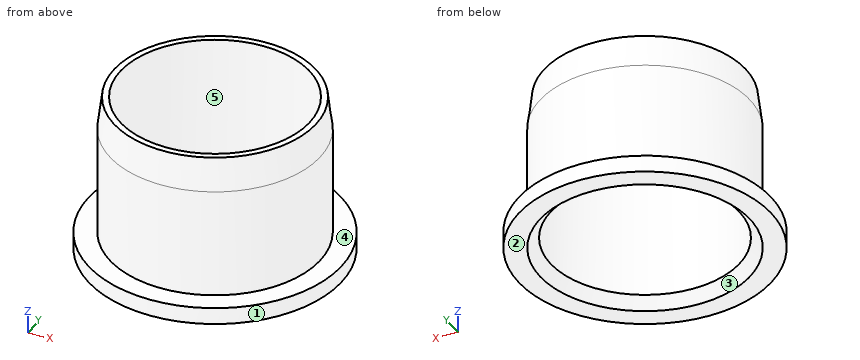
from build123d import *

# Parameters (mm, degrees)
F1_R     = 15.04
F1_R_2   = 12.5
F1_R_3   = 11.25
F2_DEPTH = 2
F3_DEPTH = 17.018
F4_SIZE2 = 4
F4_SIZE  = 0.5
F5_SIZE  = 1.25


with BuildPart() as f2:
    # F1 (on Top) → F2 (new body)
    with BuildSketch(Plane.XY):
        Circle(F1_R)
        Circle(F1_R_2, mode=Mode.SUBTRACT)
        Circle(F1_R_2)
        Circle(F1_R_3, mode=Mode.SUBTRACT)
    extrude(amount=-F2_DEPTH)

    # F1 (on Top) → F3 (join)
    with BuildSketch(Plane.XY):
        Circle(F1_R_2)
        Circle(F1_R_3, mode=Mode.SUBTRACT)
    extrude(amount=F3_DEPTH)

    # F4
    f4_edges = [f2.edges().sort_by_distance(p)[0] for p in [
        (-12.5, 0, 17.018),
    ]]
    f4_side = f2.faces().sort_by_distance((-12.146447, 0, 17.018))[0]
    chamfer(f4_edges, length=F4_SIZE, length2=F4_SIZE2, reference=f4_side)

    # F5
    f5_edges = [f2.edges().sort_by_distance(p)[0] for p in [
        (-11.25, 0, -2),
    ]]
    chamfer(f5_edges, length=F5_SIZE)


solid = f2.part
Work out the finished part from the listing and answer in its coordinate system (mm). Face numbers are marked on the shaded views. A direction names the side the tool comes from. Coordinates: 2 decimals unless noted, no trailing zeros. Write each loop counter-clockwise with the first axis right and the second up, starting at its lowest first coordinate (ties: lowest second). Pieces come first, ordered by that corner, then holes. Notation, with made-up numbers: M 57.25,36.25 L 76.25,36.25 A20 ccw 76.25,44.25 Z; hole C -7,44.5 d6. An arc over 180 degrees is marked long. Write item = value, one per line.
1. Determine the mould class of the marked faces 1, 2 and 3 for opening direction X: released by +X, released by -X, zero draft, split by the parting line, or undercut.
Solution:
face_1 = split by the parting line
face_2 = zero draft
face_3 = undercut
2. Straight lines are drawn through the part: line 1 (Y direction, x = 0, z = 6); line 2 (Y direction, x = 9, z = 1); line 3 (X direction, y = -8, z = 8). For each, find the intervals that lie inside material, in ascending order. Write a range as from..to.
Solution:
line_1 = -12.5..-11.25, 11.25..12.5
line_2 = -8.67..-6.75, 6.75..8.67
line_3 = -9.6..-7.91, 7.91..9.6
3. For the marked faces 4 and 5, determine the directions among +Z, -Z, +X, -X, +Y, -Y from which every point of the face is accessible in a straight line to the end or side of a thin tool.
Solution:
face_4 = +Z
face_5 = +Z, -Z
4. The part is cut by section C-C (z = 12). Determine the outline of the cut face in (x, y), then the cut area to 3 significant figures.
Solution:
outline = C 0,0 d25; hole C 0,0 d22.5
area = 93.3 mm2
5. Flat-ended cylindrical pins translate along their axes: pin 1 (1.5 mm diameter, centred on y = 7.5, z = 14.5, fed in from -X); pin 2 (6 mm diameter, centred on y = -6.5, z = 4.5, fed in from -X); pin 3 (1.5 mm diameter, centred on x = 2, z = 9, fed in from +Y). Find the tip coordinate at first contact, or state that the pin passes through.
Solution:
pin_1 = -10.31
pin_2 = -12
pin_3 = 12.44
6. The part is cut by section A-A (x = 0). Determine the outline of the cut face in (y, z).
Solution:
outline = M -15.04,-2 L -12.5,-2 L -11.25,-0.75 L -11.25,17.02 L -12,17.02 L -12.5,13.02 L -12.5,0 L -15.04,0 Z; M 11.25,-0.75 L 12.5,-2 L 15.04,-2 L 15.04,0 L 12.5,0 L 12.5,13.02 L 12,17.02 L 11.25,17.02 Z
